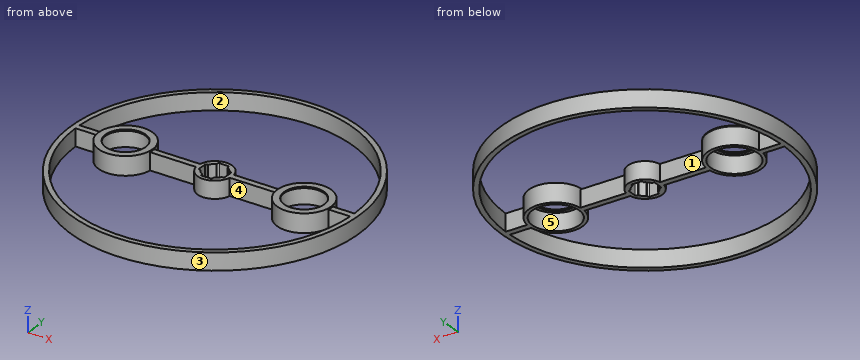
Autodesk Inventor part; units mm, degrees
ref_plane "YZ Plane" through (0, 0, 0) normal (1, 0, 0) x (0, 1, 0)
ref_plane "XZ Plane" through (0, 0, 0) normal (0, 1, 0) x (-1, 0, 0)
ref_plane "XY Plane" through (0, 0, 0) normal (0, 0, 1) x (1, 0, 0)
sketch "Sketch1" plane through (0, 0, 0) normal (0, 0, 1) x (1, 0, 0)
  circle A0 centre (0, 0) radius 40
  circle A1 centre (0, 0) radius 41.5
  circle A2 centre (0, 0) radius 3.5
  circle A3 centre (0, 0) radius 5
  circle A4 centre (26, 0) radius 6.8
  circle A5 centre (26, 0) radius 7.8
  line L0 (0, 0) -> (43.8957, 0) construction
  line L1 (4.9183, 0.9) -> (18.2521, 0.9)
  line L2 (33.7479, 0.9) -> (39.9899, 0.9)
  line L3 (4.9183, -0.9) -> (18.2521, -0.9)
  line L4 (33.7479, -0.9) -> (39.9899, -0.9)
  line L5 (-4.9183, -0.9) -> (-18.2521, -0.9)
  line L6 (-4.9183, 0.9) -> (-18.2521, 0.9)
  circle A6 centre (-26, 0) radius 7.8
  circle A7 centre (-26, 0) radius 6.8
  line L7 (-33.7479, 0.9) -> (-39.9899, 0.9)
  line L8 (-33.7479, -0.9) -> (-39.9899, -0.9)
  line L9 (1.2333, -3.7857) -> (-1.2333, -3.7857)
  line L10 (-1.6333, -3.3857) -> (-1.6333, 3.3857)
  line L11 (-1.2333, 3.7857) -> (1.2333, 3.7857)
  line L12 (1.6333, 3.3857) -> (1.6333, -3.3857)
  line L13 (1.6333, -3.7857) -> (-1.6333, 3.7857) construction
  line L14 (-1.6333, -3.7857) -> (1.6333, 3.7857) construction
  arc A8 (-1.2333, 3.7857) -> (-1.6333, 3.3857) centre (-1.2333, 3.3857) ccw
  arc A9 (1.6333, 3.3857) -> (1.2333, 3.7857) centre (1.2333, 3.3857) ccw
  arc A10 (1.2333, -3.7857) -> (1.6333, -3.3857) centre (1.2333, -3.3857) ccw
  arc A11 (-1.6333, -3.3857) -> (-1.2333, -3.7857) centre (-1.2333, -3.3857) ccw
  line L15 (3.3857, -1.6333) -> (-3.3857, -1.6333)
  line L16 (-3.7857, -1.2333) -> (-3.7857, 1.2333)
  line L17 (-3.3857, 1.6333) -> (3.3857, 1.6333)
  line L18 (3.7857, 1.2333) -> (3.7857, -1.2333)
  line L19 (3.7857, -1.6333) -> (-3.7857, 1.6333) construction
  line L20 (-3.7857, -1.6333) -> (3.7857, 1.6333) construction
  arc A12 (-3.3857, 1.6333) -> (-3.7857, 1.2333) centre (-3.3857, 1.2333) ccw
  arc A13 (3.7857, 1.2333) -> (3.3857, 1.6333) centre (3.3857, 1.2333) ccw
  arc A14 (3.3857, -1.6333) -> (3.7857, -1.2333) centre (3.3857, -1.2333) ccw
  arc A15 (-3.7857, -1.2333) -> (-3.3857, -1.6333) centre (-3.3857, -1.2333) ccw
  point P0 (-4.9183, -0.9)
  point P1 (4.9183, -0.9)
  point P2 (-1.6333, -3.0955)
  point P3 (-1.6333, 3.0955)
  point P4 (1.6333, 3.0955)
  point P5 (1.6333, -3.0955)
  point P6 (-4.9183, 0.9)
  point P7 (-33.7479, 0.9)
  point P8 (-3.0955, -1.6333)
  point P9 (-3.0955, 1.6333)
  point P10 (3.0955, 1.6333)
  point P11 (3.0955, -1.6333)
  dimension "d0" = 80
  dimension "d3" = 10
  dimension "d1" = 83
  dimension "d2" = 7
  dimension "d4" = 13.6
  dimension "d5" = 26
  dimension "d6" = 15.6
  dimension "d10" = 0.9
  dimension "d11" = 0.9
  dimension "d14" = 360
  dimension "d16" = 7.5714
  dimension "d17" = 3.2667
  dimension "d18" = 0.4
  dimension "d29" = 7.5714
  dimension "d30" = 3.2667
  dimension "d31" = 0.4
extrude "Extrusion1" add sketch "Sketch1" along normal blind 5 contours A0 L4 A5 L2 | L7 A6 L8 A0 | A5 | A6 | A5 L3 A3 L1 | L6 A3 L5 A6 | A3 | A1
sketch "Sketch3" plane through (0, 0, 5) normal (0, 0, 1) x (1, 0, 0)
  circle A0 centre (26, 0) radius 6.8
  circle A1 centre (26, 0) radius 5.8
  circle A2 centre (26, 0) radius 7.8
  point P0 (0, 0)
  dimension "d32" = 11.6
  dimension "d33" = 15.6
extrude "Extrusion3" add sketch "Sketch3" along normal blind 0.4 contours A0 | A2
pattern_circular "Circular Pattern1" count 2 over 360 about axis through (0, 0, 0) along (0, 0, 1) of "Extrusion3"
equation "\"d0\" = D_yttreRing_i"
equation "\"d3\" = D_axel + d_axelRing"
equation "\"d1\" = D_yttreRing_i + d_yttreRing"
equation "\"d2\" = D_axel"
equation "\"d4\" = D_magnet + d_toleransMagnetHållarRing"
equation "\"d6\" = d_toleransMagnetHållarRing + D_magnet + d_magnetHållarRing"
equation "\"d11\" = 0.5 * d_stöttor"
equation "\"d18\" = r_filletAxel"
equation "\"d31\" = r_filletAxel"
equation "\"d19\" = h_höjdMagnetRotor"
equation "\"d32\" = D_magnet - d_magnetSkydd"
equation "\"d33\" = d_toleransMagnetHållarRing + D_magnet + d_magnetHållarRing"
equation "\"d34\" = h_magnetSkydd"
equation "\"D_yttreRing_i\" = 80"
equation "\"d_yttreRing\" = 3"
equation "\"D_magnet\" = 13"
equation "\"D_axel\" = 7"
equation "\"d_axelRing\" = 3"
equation "\"h_höjdMagnetRotor\" = 5"
equation "\"d_stöttor\" = 1.8"
equation "\"d_toleransMagnetHållarRing\" = 0.6"
equation "\"d_magnetHållarRing\" = 2"
equation "\"l_magnetHållarRingFrånOrigo\" = 26"
equation "\"r_filletAxel\" = 0.4"
equation "\"h_magnetSkydd\" = 0.4"
equation "\"d_magnetSkydd\" = 1.4"
properties part number "Magnet_rotor_parametriserad_02"
Build history of the part. All positions in model axes, mm. Face numbers are marked on the shaded views. A direction names the side the tool comes from. Round coordinates to 2 decimals unless told otherwise and drop trailing zeros. Write each loop counter-clockwise with the first axis right and the second up, starting at its lowest first coordinate (ties: lowest second). Pieces come first, ordered by that corner, then holes. Notation, with made-up numbers: (-10.75, -3.5) - (39.25, -3.5) arc R19 cw to (39.25, 28.5) - close; hole circle Ø1 at (73.25, 39.5). An arc over 180 degrees is marked (long way). Write each question's results on one line, items separated by ' | '. Start each with the question number.
Item 1: Saw through at C-C (x = -26). Write the cut outline in (y, z).
Item 2: Saw through at D-D (y = -17). Write the cut outline in (x, z).
Item 3: Wall check: L1, parallel to Y at x = 35, z = 1.9; L2, parallel to Y at x = 26, z = 4.05; L3, parallel to X at y = 0.5, z = 3.5. Give the ranges that are in metal, low to high. Write a range as [from, to].
Item 4: Saw through at A-A (x = 0). Write the cut outline in (y, z), and give its area (3 significant figures).
Item 5: Which spindle directions (+Z, -Z, +X, -X, +Y, -Y) get a long thin tool onto all of the face, cutting with end or side? Do the marked faces 4 and 5. Say none if no direction does.
Item 6: Mould opens along Y. For the marked faces 1, 2 and 3 say: pulls with the +Y half, pulls with the -Y half, needs draft (parallel to the pull), parting line crosses it, or undercut.
Item 7: Saw through at B-B (y = 27). Write the cut outline in (x, z).
Item 8: Drop flat-ended pins along their axis: P1, Ø0.7, axis at x = 0, z = 1.5, coming from the -Y side; P2, Ø9.5, axis at x = -26, y = 0, coming from the +Z side; P3, Ø17.5, axis at x = -26, y = 0, coming from the +Z side; P4, Ø1.5, axis at x = -35.5, z = 3.5, coming from the -Y side. Give the stop position or say it passes through.
Results are:
1) outline: (-32.35, 0) - (-30.4, 0) - (-30.4, 5) - (-32.35, 5) - close; (-7.8, 0) - (-6.8, 0) - (-6.8, 5) - (-5.8, 5) - (-5.8, 5.4) - (-7.8, 5.4) - close; (5.8, 5) - (6.8, 5) - (6.8, 0) - (7.8, 0) - (7.8, 5.4) - (5.8, 5.4) - close; (30.4, 0) - (32.35, 0) - (32.35, 5) - (30.4, 5) - close
2) outline: (-37.86, 0) - (-36.21, 0) - (-36.21, 5) - (-37.86, 5) - close; (36.21, 0) - (37.86, 0) - (37.86, 5) - (36.21, 5) - close
3) L1: y = [-22.3, -19.36], [-0.9, 0.9], [19.36, 22.3] | L2: y = [-32.35, -30.4], [-7.8, -6.8], [6.8, 7.8], [30.4, 32.35] | L3: x = [-41.5, -32.78], [-19.22, -3.79], [3.79, 19.22], [32.78, 41.5]
4) outline: (-41.5, 0) - (-40, 0) - (-40, 5) - (-41.5, 5) - close; (-5, 0) - (-3.79, 0) - (-3.79, 5) - (-5, 5) - close; (3.79, 0) - (5, 0) - (5, 5) - (3.79, 5) - close; (40, 0) - (41.5, 0) - (41.5, 5) - (40, 5) - close | area: 27.1 mm²
5) face 4: +Z, -Z | face 5: -Z
6) face 1: undercut | face 2: undercut | face 3: parting line crosses it
7) outline: (-31.52, 0) - (-29.51, 0) - (-29.51, 5) - (-31.52, 5) - close; (29.51, 0) - (31.52, 0) - (31.52, 5) - (29.51, 5) - close
8) P1: stops at y = -41.5 | P2: passes through | P3: stops at z = 5.4 | P4: stops at y = -22.69
